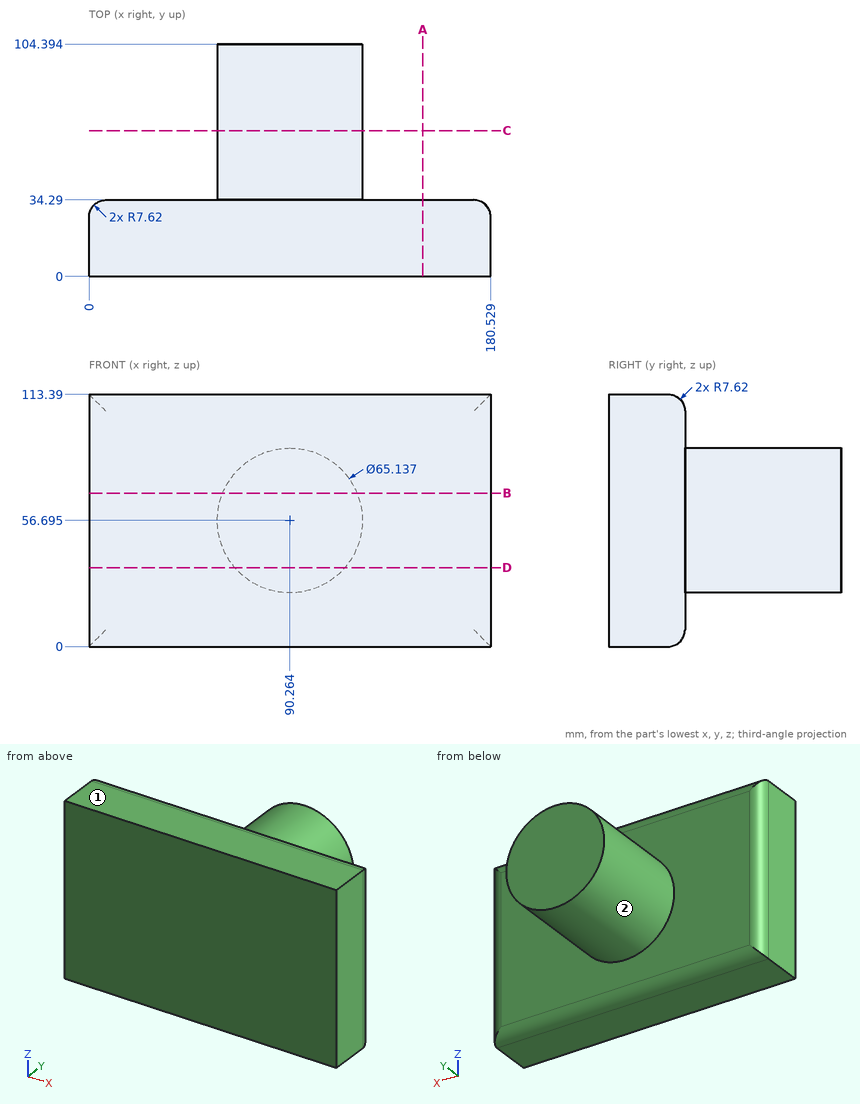
Geometry check sheet. Reference: drawing and pictorial views, mm from the part's lowest x, y, z. A direction names the side the tool comes from. Coordinates: 2 decimals unless noted, no trailing zeros. Order: outer loops, then holes, each group sorted by start corner. A loop starts at its lowest first (then second) coordinate and runs counter-clockwise, first axis right, second up. Notation, with made-up numbers: (53, -37) -> (84, -37) arc R5 cw to (84, -33) -> close; hole circle Ø11 at (-24.75, -27). An arc over 180 degrees is marked (long way). Put each result on its own line as item: value. Start each with the question number.
1) Cross-section at B-B (z = 69). Enter the section's corners in (x, y).
2) Go/stop test with flat-tipped pins: pin 1 (4 mm diameter, centred on x = 161.5, y = 33.5, fed in from +Z) (1 decimal); pin 2 (8 mm diameter, centred on y = 74.5, z = 79, fed in from +X); pin 3 (2 mm diameter, centred on x = 142, y = 33.5, fed in from +Z) (1 decimal). Record where each tip stops, or that it passes through.
3) Cross-section at C-C (y = 65.5). Enter the section's corners in (x, z) (1 decimal).
4) Tool access check on the marked faces 1 and 2. Record the directions out of +Z, -Z, +X, -X, +Y, -Y that give a thin tool (end or side, any length) a straight path to the whole face; none if there is none.
5) Cross-section at A-A (x = 150). Enter the section's corners in (y, z).
6) Cross-section at D-D (z = 35.5). Enter the section's corners in (x, y) (1 decimal).
7) Material ranges on L1, parallel to Y at x = 113.5, z = 103.5; L2, parallel to X at y = 81, z = 28 (1 decimal); L3, parallel to X at y = 30, z = 6.5 (1 decimal), recorded low to high.
Geometry check:
1. outline: (0, 0) -> (180.53, 0) -> (180.53, 26.67) arc R7.62 ccw to (172.91, 34.29) -> (120.42, 34.29) -> (120.42, 104.39) -> (60.11, 104.39) -> (60.11, 34.29) -> (7.62, 34.29) arc R7.62 ccw to (0, 26.67) -> close
2. pin 1: stops at z = 111.7
2. pin 2: stops at x = 117.2
2. pin 3: stops at z = 110.7
3. outline: circle Ø65.1 at (90.3, 56.7)
4. face 1: +Z, +X, -X, +Y, -Y
4. face 2: +Y
5. outline: (0, 0) -> (26.67, 0) arc R7.62 ccw to (34.29, 7.62) -> (34.29, 105.77) arc R7.62 ccw to (26.67, 113.39) -> (0, 113.39) -> close
6. outline: (0, 0) -> (180.5, 0) -> (180.5, 26.7) arc R7.6 ccw to (172.9, 34.3) -> (115, 34.3) -> (115, 104.4) -> (65.5, 104.4) -> (65.5, 34.3) -> (7.6, 34.3) arc R7.6 ccw to (0, 26.7) -> close
7. L1: y = 0 to 34.29
7. L2: x = 74.9 to 105.7
7. L3: x = 0.8 to 179.8
